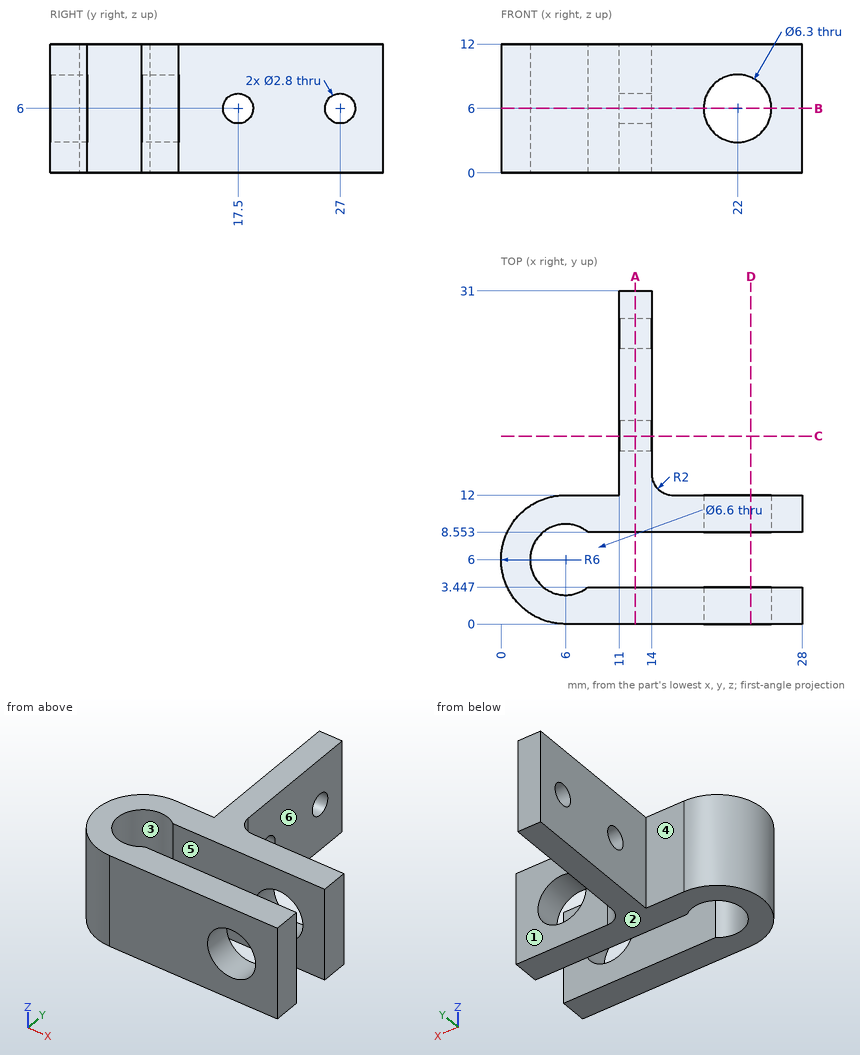
Drawing for the job (mm, zero at the part's lowest x, y, z). A direction names the side the tool comes from. Round coordinates to 2 decimals unless told otherwise and drop trailing zeros. Order: outer loops, then holes, each group sorted by start corner. A loop starts at its lowest first (then second) coordinate and runs counter-clockwise, first axis right, second up. Notation, with made-up numbers: M 37,0.25 L 90,0.25 A21 ccw 90,32.25 Z; hole C 65.25,13 d1. An arc over 180 degrees is marked long. Use one line per item in the form item = value.
Q1. Saw through at C-C on y = 17.5. Give the cut face in (x, z).
Recorded:
outline = M 11,0 L 14,0 L 14,4.6 L 11,4.6 Z; M 11,7.4 L 14,7.4 L 14,12 L 11,12 Z
Q2. Saw through at B-B on z = 6. State how many separate pieces and enclosed holes the cut face has, then the cut area to 3 significant figures.
Recorded:
separate_pieces = 5
enclosed_holes = 0
area = 187 mm^2
Q3. Which spindle directions (+Z, -Z, +X, -X, +Y, -Y) get a long thin tool onto all of the face, cutting with end or side? Do the marked faces 4, 5 and 6. Say none if no direction does.
Recorded:
face_4 = +Z, -Z, -X, +Y
face_5 = +Z, -Z, +X
face_6 = +Z, -Z, +X, +Y
Q4. Saw through at A-A on x = 12.5. Give the cut face in (y, z).
Recorded:
outline = M 0,0 L 3.45,0 L 3.45,12 L 0,12 Z; M 8.55,0 L 31,0 L 31,12 L 8.55,12 Z; hole C 17.5,6 d2.8; hole C 27,6 d2.8
Q5. Two-plate mould, pull along Y, no slides. Class the marked faces 1, 2 and 3: +Y half, -Y half, draft (parallel to the pull), parting line (faces both ways), or undercut.
Recorded:
face_1 = +Y half
face_2 = draft
face_3 = undercut
Q6. Flat gauge pins, fed straight in: P1, Ø2.5, axis at y = 17.5, z = 6, coming from the -X side; P2, Ø7, axis at x = 22, z = 6, coming from the +Y side; P3, Ø6, axis at y = 28, z = 5.5, coming from the -X side. Where does each tip first touch, or does it go through?
Recorded:
P1 = through
P2 = 12
P3 = 11
Q7. Saw through at D-D on x = 23.25. Give the cut face in (y, z).
Recorded:
outline = M 0,0 L 3.45,0 L 3.45,3.11 L 0,3.11 Z; M 0,8.89 L 3.45,8.89 L 3.45,12 L 0,12 Z; M 8.55,0 L 12,0 L 12,3.11 L 8.55,3.11 Z; M 8.55,8.89 L 12,8.89 L 12,12 L 8.55,12 Z
Q8. Probe L1, parallel to Y at x = 12.15, z = 6; L2, parallel to Y at x = 13.75, z = 5.5; L3, parallel to Z at x = 22, y = 2.3. List the from-to ranges inside material, lowest first.
Recorded:
L1 = 0 to 3.45, 8.55 to 16.1, 18.9 to 25.6, 28.4 to 31
L2 = 0 to 3.45, 8.55 to 16.19, 18.81 to 25.69, 28.31 to 31
L3 = 0 to 2.85, 9.15 to 12
